```python
from build123d import *

# Parameters (mm, degrees)
BOSS_EXTRUDE1_DEPTH = 5
FILLET1_R           = 0.6
FILLET2_R           = 0.2


with BuildPart() as part:
    # Sketch1 → Boss-Extrude1 (new body)
    with BuildSketch(Plane(origin=(0, 0, 0), x_dir=(1, 0, 0), z_dir=(0, 1, 0))):
        Polygon((-5, 0), (5, 0), (5, -4.8), (1, -4.8), (1, -3.6), (3.8, -3.6), (3.8, -1.2), (-3.8, -1.2), (-3.8, -3.6), (-1, -3.6), (-1, -4.8), (-5, -4.8), align=None)
    extrude(amount=BOSS_EXTRUDE1_DEPTH)

    # Fillet1
    fillet1_edges = [part.edges().sort_by_distance(p)[0] for p in [
        (-5, 2.5, 0),
        (5, 2.5, 0),
        (5, 2.5, 4.8),
        (1, 2.5, 4.8),
        (1, 2.5, 3.6),
        (-1, 2.5, 3.6),
        (-1, 2.5, 4.8),
        (-5, 2.5, 4.8),
    ]]
    fillet(fillet1_edges, radius=FILLET1_R - 0.0001)  # a hair under: the kernel refuses the full size

    # Fillet2
    fillet2_edges = [part.edges().sort_by_distance(p)[0] for p in [
        (3.8, 2.5, 3.6),
        (3.8, 2.5, 1.2),
        (-3.8, 2.5, 1.2),
        (-3.8, 2.5, 3.6),
    ]]
    fillet(fillet2_edges, radius=FILLET2_R)


solid = part.part
```
Geometry: final body of the model. Coordinates: model frame, mm. A direction names the side the tool comes from. Coordinates: 2 decimals unless noted, no trailing zeros. Order: outer loops, then holes, each group sorted by start corner. A loop starts at its lowest first (then second) coordinate and runs counter-clockwise, first axis right, second up. Notation, with made-up numbers: M 4,9.5 L 9,9.5 A22 ccw 9,17.5 Z; hole C -15,-12 d5. An arc over 180 degrees is marked long. Answer in a Markdown table with one row per item. Add a question column.
Q1. Section query A-A on z = 1.85. Return the cut outline in (x, y), and give its area (3 significant figures).
Q2. Section query C-C on x = 2.25. Return the cut outline in (y, z).
Q3. Mould query, pull axis X, two halves, no side actions, for faces 1 (the flat face through (0, 0, 1)), 2 (the flat face through (3.8, 2, 2)), 3 (the flat face through (5, 2, 2)), 4 (the flat face through (-3.8, 2, 2)). Classes: released by +X, released by -X, zero draft, split by the parting line, or undercut.
Q4. Contact query for a flat-ended pin moving along its axis: P1, Ø1.5, axis at x = 0.5, y = 1.5, coming from the +Z side. Output: stop coordinate, or through.
Q5. Reachability of faces 5 (the flat face through (0, 5, 1)), 6 (the flat face through (0, 2, 1.2)) from +Z, -Z, +X, -X, +Y, -Y: full face, straight path, thin tool, end or side. Return the list, or none.
Q6. Section query D-D on x = -0.5. Return the cut outline in (y, z).
Q7. Line query: L1, parallel to Z at x = 2, y = 1.05; L2, parallel to X at y = 3.55, z = 2.15; L3, parallel to X at y = 2.95, z = 4.25. Output: solid intervals per line, ascending.
Completed:
| question | item | result |
|---|---|---|
| 1 | outline | M -5,0 L -3.8,0 L -3.8,5 L -5,5 Z; M 3.8,0 L 5,0 L 5,5 L 3.8,5 Z |
| 1 | area | 12.0 mm2 |
| 2 | outline | M 0,0 L 5,0 L 5,1.2 L 0,1.2 Z; M 0,3.6 L 5,3.6 L 5,4.8 L 0,4.8 Z |
| 3 | face 1 | zero draft |
| 3 | face 2 | undercut |
| 3 | face 3 | released by +X |
| 3 | face 4 | undercut |
| 4 | P1 | stops at z = 4.69 |
| 5 | face 5 | +Z, -Z, +X, -X, +Y |
| 5 | face 6 | +Y, -Y |
| 6 | outline | M 0,0 L 5,0 L 5,1.2 L 0,1.2 Z |
| 7 | L1 | z = 0 to 1.2, 3.6 to 4.8 |
| 7 | L2 | x = -5 to -3.8, 3.8 to 5 |
| 7 | L3 | x = -5 to -1, 1 to 5 |
